The listing builds one solid part. Answer for the finished solid, in the listing's coordinates (mm). Coordinates: 2 decimals unless noted, no trailing zeros. Loops run counter-clockwise (first coordinate to the right, second up) from the corner with the lowest first, then second, coordinate; pieces in that order, holes last. Notation, with made-up numbers: M 26.5,-1.5 L 54.5,-1.5 A22 ccw 54.5,15.5 Z; hole C -30,15.5 d4. An arc over 180 degrees is marked long. Return JSON: item names as keys, results as strings. Group by question number.
1. Section A-A (y = 279) is taken. Write down the section's boundary in (x, z).
2. Section C-C (z = 2.55) is taken. Count the separate pieces of the cut face and the enclosed holes in it, then the cut area to 3 significant figures.
3. Straight lines are drawn through the part: L1, parallel to Y at x = 238, z = 2.2; L2, parallel to Y at x = 179.5, z = 2.4; L3, parallel to Y at x = 161, z = 1.4. For each, find the intervals that lie inside material, in ascending order. Write a range as from..to.
4. Section D-D (y = 51) is taken. Write down the section's boundary in (x, z).
5. Given P1, Ø2.5, axis at y = 183, z = 2, coming from the -X side; P2, Ø1.5, axis at y = 273, z = 3.5, coming from the -X side; P3, Ø2.5, axis at y = 200.5, z = 3, coming from the +X side, each flat-ended and moving along its own axis, determine where each tip first touches the part or whether it passes through.
6. Section B-B (x = -39) is taken. Write down the section's boundary in (y, z), then the cut area to 3 significant figures.
```python
from build123d import *

# Parameters (mm, degrees)
SKETCH1_W           = 66
SKETCH1_H           = 50
SKETCH1_R           = 1
BOSS_EXTRUDE1_DEPTH = 5
SKETCH2_R           = 1
CUT_EXTRUDE1_DEPTH  = 388.996134001
SKETCH3_R           = 1
SKETCH3_W           = 20
SKETCH3_H           = 5
CUT_EXTRUDE2_DEPTH  = 388.996134001
SKETCH4_W           = 5
SKETCH4_H           = 5
CUT_EXTRUDE3_DEPTH  = 388.996134001


with BuildPart() as part:
    # Sketch1 → Boss-Extrude1 (new body)
    # profile 1 of 3: a face of its own
    with BuildSketch(Plane.XY):
        with Locations((-33, 85)):
            Rectangle(SKETCH1_W, SKETCH1_H)
    # profile 2 of 3: a face of its own
    with BuildSketch(Plane.XY):
        Polygon((0, 60), (0, 0), (180, 0), (180, 60), (180, 110), (180, 300), (130, 300), (130, 150), (50, 150), (50, 300), (0, 300), (0, 110), align=None)
        with Locations((19, 117.5)):
            Circle(SKETCH1_R, mode=Mode.SUBTRACT)
        with Locations((38, 117.5)):
            Circle(SKETCH1_R, mode=Mode.SUBTRACT)
        with Locations((19, 134)):
            Circle(SKETCH1_R, mode=Mode.SUBTRACT)
        with Locations((38, 134)):
            Circle(SKETCH1_R, mode=Mode.SUBTRACT)
        with Locations((142, 117.5)):
            Circle(SKETCH1_R, mode=Mode.SUBTRACT)
        with Locations((161, 117.5)):
            Circle(SKETCH1_R, mode=Mode.SUBTRACT)
        with Locations((142, 134)):
            Circle(SKETCH1_R, mode=Mode.SUBTRACT)
        with Locations((161, 134)):
            Circle(SKETCH1_R, mode=Mode.SUBTRACT)
    # profile 3 of 3: a face of its own
    with BuildSketch(Plane.XY):
        with Locations((213, 85)):
            Rectangle(SKETCH1_W, SKETCH1_H)
    extrude(amount=BOSS_EXTRUDE1_DEPTH)

    # Sketch2 → Cut-Extrude1 (cut, through all)
    with BuildSketch(Plane.XY.offset(5)):
        with Locations((-58, 103)):
            Circle(SKETCH2_R)
        with Locations((-58, 67)):
            Circle(SKETCH2_R)
        with Locations(Location((238, 67, 0), (0, 0, 180))):
            Circle(SKETCH2_R)
        with Locations(Location((238, 103, 0), (0, 0, 180))):
            Circle(SKETCH2_R)
    extrude(amount=-CUT_EXTRUDE1_DEPTH, mode=Mode.SUBTRACT)

    # Sketch3 → Cut-Extrude2 (cut, through all)
    with BuildSketch(Plane.XY.offset(5)):
        with Locations((19, 77)):
            Circle(SKETCH3_R)
        with Locations((19, 99.5)):
            Circle(SKETCH3_R)
        with Locations(Location((161, 77, 0), (0, 0, 180))):
            Circle(SKETCH3_R)
        with Locations(Location((161, 99.5, 0), (0, 0, 180))):
            Circle(SKETCH3_R)
        with Locations((-6, 90)):
            Rectangle(SKETCH3_W, SKETCH3_H)
        with Locations((186, 90)):
            Rectangle(SKETCH3_W, SKETCH3_H)
    extrude(amount=-CUT_EXTRUDE2_DEPTH, mode=Mode.SUBTRACT)

    # Sketch4 → Cut-Extrude3 (cut, through all)
    with BuildSketch(Plane.XY.offset(5)):
        with Locations((2.5, 272.5)):
            Rectangle(SKETCH4_W, SKETCH4_H)
        with Locations((47.5, 272.5)):
            Rectangle(SKETCH4_W, SKETCH4_H)
        with Locations((132.5, 272.5)):
            Rectangle(SKETCH4_W, SKETCH4_H)
        with Locations((177.5, 272.5)):
            Rectangle(SKETCH4_W, SKETCH4_H)
    extrude(amount=-CUT_EXTRUDE3_DEPTH, mode=Mode.SUBTRACT)


solid = part.part
```
Worked out:
{
 "1": {"outline": "M 0,0 L 50,0 L 50,5 L 0,5 Z; M 130,0 L 180,0 L 180,5 L 130,5 Z"},
 "2": {"separate pieces": "1", "enclosed holes": "18", "area": "48,200 mm^2"},
 "3": {"L1": "60..66, 68..102, 104..110", "L2": "0..87.5, 92.5..270, 275..300", "L3": "0..76, 78..98.5, 100.5..116.5, 118.5..133, 135..300"},
 "4": {"outline": "M 0,0 L 180,0 L 180,5 L 0,5 Z"},
 "5": {"P1": "x = 0", "P2": "x = 5", "P3": "x = 180"},
 "6": {"outline": "M 60,0 L 110,0 L 110,5 L 60,5 Z", "area": "250 mm^2"}
}
